Read the model definition and answer for the solid it produces. Units are mm, in the model's axes. Face numbers are marked on the shaded views. A direction names the side the tool comes from. Coordinates: 2 decimals unless noted, no trailing zeros. Loops run counter-clockwise (first coordinate to the right, second up) from the corner with the lowest first, then second, coordinate; pieces in that order, holes last.
Q1. Section D-D (y = 10.5) is taken. Give the vertices of the cut face in (x, z), then the cut area to 3 significant figures.
Q2. Section C-C (y = 7.5) is taken. Give the vertices of the cut face in (x, z), then the cut area to 3 significant figures.
Q3. Straight lines are drawn through the part: line 1 (X direction, y = 12.75, z = 3.5); line 2 (X direction, y = 9.75, z = 1); line 3 (Y direction, x = 1, z = 2.25). For each, find the intervals that lie inside material, in ascending order.
Q4. Section A-A (z = 4.25) is taken. Give the vertices of the cut face in (x, y) (1 decimal).
Q5. Section B-B (x = -0.5) is taken. Give the vertices of the cut face in (y, z).
Q6. The mould has two halves that part along X. Classify the marked faces 1, 2 and 3: pulls with the +X half, pulls with the -X half, needs draft (parallel to the pull), parting line crosses it, or undercut.
Q7. Flat-ended cylindrical pins translate along their axes: P1, Ø2.5, axis at y = 13.5, z = 3, coming from the +X side; P2, Ø1.1, axis at y = 12.5, z = 2.5, coming from the +X side; P3, Ø4.5, axis at x = -0.5, z = 5.5, coming from the -Y side; P4, Ø4, axis at y = 13, z = 3.5, coming from the -X side. Find the tip coordinate at first contact, or state that the pin passes through.
Q8. Which of the six approach directions +Z, -Z, +X, -X, +Y, -Y give full straight-line access (tool end or side, diameter ignored) to the marked faces 4 and 5?
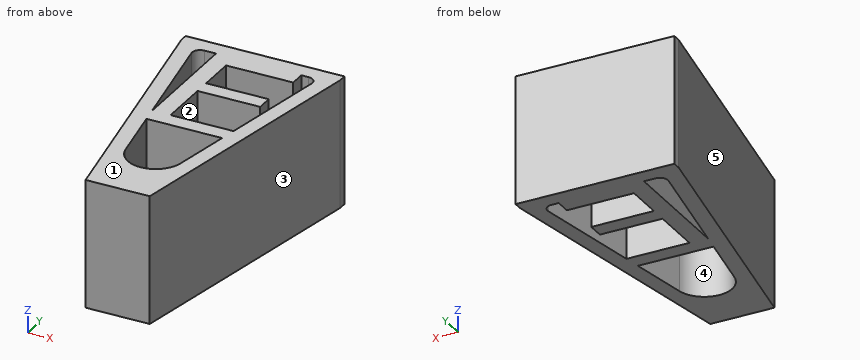
Autodesk Inventor part; units mm, degrees
ref_plane "YZ Plane" through (0, 0, 0) normal (1, 0, 0) x (0, 1, 0)
ref_plane "XZ Plane" through (0, 0, 0) normal (0, 1, 0) x (-1, 0, 0)
ref_plane "XY Plane" through (0, 0, 0) normal (0, 0, 1) x (1, 0, 0)
sketch "Sketch1" plane through (0, 0, 0) normal (0, 0, 1) x (1, 0, 0)
  line L0 (0, 0) -> (0, 17.2417) construction
  line L1 (0, 17.2417) -> (-4.952, 17.2417)
  line L2 (-4.952, 17.2417) -> (-4.952, 16.7417)
  line L3 (-4.952, 16.7417) -> (-2, 0)
  line L4 (-2, 0) -> (0, 0)
  line L5 (0, 17.2417) -> (4.952, 17.2417)
  line L6 (4.952, 17.2417) -> (4.952, 16.7417)
  line L7 (4.952, 16.7417) -> (2, 0)
  line L8 (2, 0) -> (0, 0)
  line L9 (-3.2526, 16.2417) -> (0.4283, 16.2417)
  line L10 (0.4283, 16.2417) -> (3.2526, 16.2417)
  line L11 (3.745, 15.6549) -> (1.7172, 4.155)
  line L12 (-1.7172, 4.155) -> (-3.745, 15.6549)
  arc A0 (-3.2526, 16.2417) -> (-3.745, 15.6549) centre (-3.2526, 15.7417) ccw
  arc A1 (3.745, 15.6549) -> (3.2526, 16.2417) centre (3.2526, 15.7417) ccw
  arc A2 (-1.7172, 4.155) -> (1.7172, 4.155) centre (0, 4.4578) ccw
  line L13 (-3.3837, 16.2973) -> (4.7039, 16.2973) construction
  line L14 (4.7039, 16.2973) -> (4.7039, 6.2973) construction
  line L15 (4.7039, 6.2973) -> (-3.3837, 6.2973) construction
  line L16 (-3.3837, 6.2973) -> (-3.3837, 16.2973) construction
  line L17 (-2.5226, 7.7973) -> (-2.5226, 16.2973)
  line L18 (-2.5226, 16.2973) -> (2.795, 16.2973)
  line L19 (2.795, 16.2973) -> (2.795, 15.2917)
  line L20 (2.795, 15.2917) -> (-1.393, 15.2917)
  line L21 (-1.393, 15.2917) -> (-1.393, 12.9635)
  line L22 (-1.393, 12.9635) -> (2.5126, 12.9635)
  line L23 (2.5126, 12.9635) -> (2.5126, 11.9578)
  line L24 (2.5126, 11.9578) -> (-1.393, 11.9578)
  line L25 (-1.393, 11.9578) -> (-1.393, 8.803)
  line L26 (-1.393, 8.803) -> (2.795, 8.803)
  line L27 (2.795, 8.803) -> (2.795, 7.7973)
  line L28 (2.795, 7.7973) -> (-2.5226, 7.7973)
  point P0 (-3.8484, 16.2417)
  point P1 (3.8484, 16.2417)
  point P2 (0, -5.5838)
  dimension "d0" = 2
  dimension "d1" = 10
  dimension "d2" = 0.5
  dimension "d3" = 17
  dimension "d4" = 1
  dimension "d7" = 0.5
extrude "Extrusion1" add sketch "Sketch1" along normal blind 8 contours L5 L6 L7 L8 L4 L3 L2 L1 | L17 L18 L19 L10 L9 | L9 L10 L19 L20 L21 L22 L23 L24 L25 L26 L11 L28 L12 L17 | L12 L28 L17 | L11 L26 L27 L28
properties part number "MainBracketE"
Numbers:
1. outline: (-3.85, 0) - (-2.84, 0) - (-2.84, 8) - (-3.85, 8) - close; (-2.52, 0) - (-1.39, 0) - (-1.39, 8) - (-2.52, 8) - close; (2.84, 0) - (3.85, 0) - (3.85, 8) - (2.84, 8) - close
1. area: 25.3 mm2
2. outline: (-3.32, 0) - (-2.31, 0) - (-2.31, 8) - (-3.32, 8) - close; (2.31, 0) - (3.32, 0) - (3.32, 8) - (2.31, 8) - close
2. area: 16.2 mm2
3. line 1: x = -4.25 to -3.23, -2.52 to 2.51, 3.23 to 4.25
3. line 2: x = -3.72 to -2.7, -2.52 to -1.39, 2.7 to 3.72
3. line 3: y = 0 to 3.03, 7.8 to 8.8, 11.96 to 12.96, 15.29 to 17.24
4. outline: (-5, 16.7) - (-2, 0) - (2, 0) - (5, 16.7) - (5, 17.2) - (-5, 17.2) - close; hole (-3.7, 15.7) - (-2.5, 8.7) - (-2.5, 16.2) - (-3.3, 16.2) arc R0.5 ccw to start; hole (-2.4, 7.8) - (-1.7, 4.2) arc R1.7 ccw to (1.7, 4.2) - (2.4, 7.8) - close; hole (-1.4, 8.8) - (2.5, 8.8) - (3.7, 15.7) arc R0.5 ccw to (3.3, 16.2) - (2.8, 16.2) - (2.8, 15.3) - (-1.4, 15.3) - (-1.4, 13) - (2.5, 13) - (2.5, 12) - (-1.4, 12) - close
5. outline: (0, 0) - (2.79, 0) - (2.79, 8) - (0, 8) - close; (7.8, 0) - (8.8, 0) - (8.8, 8) - (7.8, 8) - close; (11.96, 0) - (12.96, 0) - (12.96, 8) - (11.96, 8) - close; (15.29, 0) - (17.24, 0) - (17.24, 8) - (15.29, 8) - close
6. face 1: needs draft
6. face 2: undercut
6. face 3: pulls with the +X half
7. P1: stops at x = 4.6
7. P2: stops at x = 4.3
7. P3: stops at y = 0
7. P4: stops at x = -4.64
8. face 4: +Z, -Z
8. face 5: +Z, -Z, -X, -Y
